Geometry: final body of the model. Coordinates: model frame, mm. A direction names the side the tool comes from. Give positions to 0.01 mm unless a question says otherwise; leave off trailing zeros. Loops run counter-clockwise (first coordinate to the right, second up) from the corner with the lowest first, then second, coordinate; pieces in that order, holes last.
from build123d import *

# Parameters (mm, degrees)
BOSS_EXTRUDE1_DEPTH = 4


with BuildPart() as part:
    # Sketch1 → Boss-Extrude1 (new body)
    with BuildSketch(Plane(origin=(0, 0, 0), x_dir=(1, 0, 0), z_dir=(0, 1, 0))):
        with BuildLine():
            Line((-4, 0), (-4, 12.5))
            Line((-4, 12.5), (-20, 12.5))
            Line((-20, 12.5), (-20, -12.5))
            Line((-20, -12.5), (20, -12.5))
            Line((20, -12.5), (20, 12.5))
            Line((20, 12.5), (4, 12.5))
            Line((4, 12.5), (4, 0))
            ThreePointArc((4, 0), (0, -4), (-4, 0))
        make_face()
    extrude(amount=BOSS_EXTRUDE1_DEPTH)


solid = part.part
Item 1: Section query A-A on z = -10.5. Return loops of the section in (x, y), plus the area to 3 significant figures.
Values follow:
outline: (-20, 0) - (-4, 0) - (-4, 4) - (-20, 4) - close; (4, 0) - (20, 0) - (20, 4) - (4, 4) - close
area: 128 mm2
Item 2: Section query B-B on y = 1.75. Return loops of the section in (x, z).
Values follow:
outline: (-20, -12.5) - (-4, -12.5) - (-4, 0) arc R4 cw to (4, 0) - (4, -12.5) - (20, -12.5) - (20, 12.5) - (-20, 12.5) - close
Item 3: Section query C-C on x = 0. Return loops of the section in (y, z).
Values follow:
outline: (0, 4) - (4, 4) - (4, 12.5) - (0, 12.5) - close
Item 4: Ray query, probe 1 along X at (y, z) = (3.4, -11.5); probe 2 along X at (y, z) = (1.4, 3.25); probe 3 along Z at (x, y) = (0, 3.7). Return the intervals inside material, ascending.
Values follow:
probe 1: x = -20 to -4, 4 to 20
probe 2: x = -20 to -2.33, 2.33 to 20
probe 3: z = 4 to 12.5
Item 5: Set-up query: faces 1 (the face through (4, 2, -6)), 2 (the face through (0, 2, 12.5)). Return all of +Z, -Z, +X, -X, +Y, -Y with unobstructed straight access to the full face (end or side cutting, diameter ignored); none if empty.
Values follow:
face 1: -Z, +Y, -Y
face 2: +Z, +X, -X, +Y, -Y
Item 6: Draft query along X for faces 3 (the face through (-5, 0, 0)), 4 (the face through (-20, 2, 0)), 5 (the face through (20, 2, 0)), 6 (the face through (-4, 2, -6)). Return one class per face: +X half, -X half, draft (parallel to the pull), parting line (faces both ways), or undercut.
Values follow:
face 3: draft
face 4: -X half
face 5: +X half
face 6: undercut
